Part model, mm, in its own coordinate system. A direction names the side the tool comes from. Round coordinates to 2 decimals unless told otherwise and drop trailing zeros. Loops run counter-clockwise (first coordinate to the right, second up) from the corner with the lowest first, then second, coordinate; pieces in that order, holes last.
1) Band-saw the part on A-A, the plane z = 5.5. Write the cut outline in (x, y).
2) Band-saw the part on C-C, the plane x = 23.5. Write the cut outline in (y, z), then the cut area to 3 significant figures.
3) Band-saw the part on D-D, the plane y = 9. Write the cut outline in (x, z).
4) Mould opens along Y. For faces 1 (the flat face through (19.5, 1, 22)), 2 (the flat face through (4, 6.5, 13)), 3 (the flat face through (13, 4.998, 22)) say: +Y half, -Y half, draft (parallel to the pull), parting line (faces both ways), or undercut.
5) Probe line 1 (X direction, y = 7.45, z = 12.7); line 2 (X direction, y = 7.5, z = 41); line 3 (Y direction, x = 18.75, z = 34.5). List the from-to ranges inside material, lowest first.
6) Drop flat-ended pins along their axis: P1, Ø1.8, axis at x = 23.5, z = 32.7, coming from the +Y side; P2, Ø0.5, axis at x = 8.5, z = 11.5, coming from the -Y side. Give the stop position or say it passes through.
7) 3-axis set-ups, long thin cutter, end or side, ignore diameter. For faces 4 (the flat face through (4, 6.5, 33)), 5 (the flat face through (8, 2.248, 22)), 6 (the flat face through (8, 3.248, 22)): which of +Z, -Z, +X, -X, +Y, -Y reach the whole face in a straight line?
8) Band-saw the part on B-B, the plane y = 4.5. Write the cut outline in (x, z).
from build123d import *

# Parameters (mm, degrees)
DODANIE_WYCI_GNI_CIE1_DEPTH    = 45.4
OTWORY_USTALAJ_CE_1_0MM1_D     = 0.8
OTWORY_USTALAJ_CE_1_0MM1_DEPTH = 6.5
OTWORY_USTALAJ_CE_1_0MM1_TIP   = 0.240344248
OTWORY_USTALAJ_CE_1_0MM2_D     = 0.8
OTWORY_USTALAJ_CE_1_0MM2_DEPTH = 6.5
OTWORY_USTALAJ_CE_1_0MM2_TIP   = 0.240344248
F_3_0MM_DOWEL_HOLE1_D          = 3
F_3_0MM_DOWEL_HOLE1_DEPTH      = 3.5


with BuildPart() as part:
    # Szkic1 → Dodanie-wyciągnięcie1 (new body)
    with BuildSketch(Plane.XY):
        Polygon((7.5, 0), (7.5, 2.247882756), (9.25, 2.247882756), (9.25, 3.247882756), (7.5, 3.247882756), (7.5, 4.997882756), (19.5, 4.997882756), (19.5, 3.247882756), (17.75, 3.247882756), (17.75, 2.247882756), (19.5, 2.247882756), (19.5, 0), (27, 0), (27, 10), (0, 10), (0, 0), align=None)
    extrude(amount=DODANIE_WYCI_GNI_CIE1_DEPTH)

    # Otwory ustalające Ø1.0mm1
    with Locations(Plane.XY.offset(45.4)):
        with Locations((13.5, 7.5)):
            Hole(OTWORY_USTALAJ_CE_1_0MM1_D / 2, depth=OTWORY_USTALAJ_CE_1_0MM1_DEPTH)
            with Locations((0, 0, -(OTWORY_USTALAJ_CE_1_0MM1_DEPTH + OTWORY_USTALAJ_CE_1_0MM1_TIP / 2))):  # 118° drill point
                Cone(0, OTWORY_USTALAJ_CE_1_0MM1_D / 2, OTWORY_USTALAJ_CE_1_0MM1_TIP, mode=Mode.SUBTRACT)

    # Otwory ustalające Ø1.0mm2
    with Locations(Plane(origin=(0, 0, 0), x_dir=(-1, 0, 0), z_dir=(0, 0, -1))):
        with Locations((-13.5, 7.5)):
            Hole(OTWORY_USTALAJ_CE_1_0MM2_D / 2, depth=OTWORY_USTALAJ_CE_1_0MM2_DEPTH)
            with Locations((0, 0, -(OTWORY_USTALAJ_CE_1_0MM2_DEPTH + OTWORY_USTALAJ_CE_1_0MM2_TIP / 2))):  # 118° drill point
                Cone(0, OTWORY_USTALAJ_CE_1_0MM2_D / 2, OTWORY_USTALAJ_CE_1_0MM2_TIP, mode=Mode.SUBTRACT)

    # Ø3.0mm Dowel Hole1
    with Locations(Plane(origin=(0, 10, 0), x_dir=(1, 0, 0), z_dir=(0, 1, 0))):
        with Locations((3.5, -32.7), (23.5, -32.7), (23.5, -12.7), (3.5, -12.7)):
            Hole(F_3_0MM_DOWEL_HOLE1_D / 2, depth=F_3_0MM_DOWEL_HOLE1_DEPTH)


solid = part.part
Reported:
1. outline: (0, 0) - (7.5, 0) - (7.5, 2.25) - (9.25, 2.25) - (9.25, 3.25) - (7.5, 3.25) - (7.5, 5) - (19.5, 5) - (19.5, 3.25) - (17.75, 3.25) - (17.75, 2.25) - (19.5, 2.25) - (19.5, 0) - (27, 0) - (27, 10) - (0, 10) - close; hole circle Ø0.8 at (13.5, 7.5)
2. outline: (0, 0) - (10, 0) - (10, 11.2) - (6.5, 11.2) - (6.5, 14.2) - (10, 14.2) - (10, 31.2) - (6.5, 31.2) - (6.5, 34.2) - (10, 34.2) - (10, 45.4) - (0, 45.4) - close
2. area: 433 mm2
3. outline: (0, 0) - (27, 0) - (27, 45.4) - (0, 45.4) - close; hole circle Ø3 at (3.5, 12.7); hole circle Ø3 at (3.5, 32.7); hole circle Ø3 at (23.5, 12.7); hole circle Ø3 at (23.5, 32.7)
4. face 1: draft
4. face 2: +Y half
4. face 3: undercut
5. line 1: x = 0 to 2, 5 to 22, 25 to 27
5. line 2: x = 0 to 13.1, 13.9 to 27
5. line 3: y = 2.25 to 3.25, 5 to 10
6. P1: stops at y = 6.5
6. P2: stops at y = 2.25
7. face 4: +Y
7. face 5: +Z, -Z, -Y
7. face 6: +Z, -Z
8. outline: (0, 0) - (7.5, 0) - (7.5, 45.4) - (0, 45.4) - close; (19.5, 0) - (27, 0) - (27, 45.4) - (19.5, 45.4) - close
